Source: CAD feature listing. Evaluate the final solid. Frame: model axes, mm. Face numbers are marked on the shaded views. A direction names the side the tool comes from. Coordinates: 2 decimals unless noted, no trailing zeros. Order: outer loops, then holes, each group sorted by start corner. A loop starts at its lowest first (then second) coordinate and runs counter-clockwise, first axis right, second up. Notation, with made-up numbers: (7, -22.5) - (41, -22.5) arc R13 ccw to (41, -18.5) - close; hole circle Ø5 at (81, -24.75). An arc over 180 degrees is marked (long way). One line per question, with ' | ' between items.
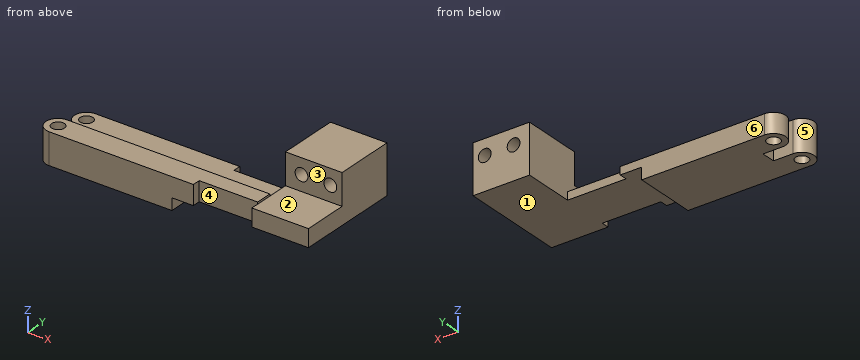
Autodesk Inventor part; units mm, degrees
ref_plane "作業平面1" through (0, 0, 5) normal (0, 0, -1) x (-1, 0, 0)
ref_plane "YZ Plane" through (0, 0, 0) normal (1, 0, 0) x (0, 1, 0)
ref_plane "XZ Plane" through (0, 0, 0) normal (0, 1, 0) x (-1, 0, 0)
sketch "スケッチ1" plane through (0, 0, 0) normal (0, 0, 1) x (1, 0, 0)
  line L0 (-3, 8) -> (3, 8)
  line L1 (3, 8) -> (3, -8)
  line L2 (3, -8) -> (-3, -8)
  line L3 (-3, -8) -> (-3, 8)
  line L4 (-3, 8) -> (3, -8) construction
  line L5 (3, 8) -> (-3, -8) construction
  line L6 (0, 8) -> (0, -8) construction
  circle A0 centre (0, 4.9) radius 1.635
  circle A1 centre (0, -4.9) radius 1.635
  line L7 (0, 4.9) -> (0, -4.9)
  line L8 (-3, 0) -> (3, 0)
  circle A2 centre (0, 4.9) radius 3.1
  circle A3 centre (0, -4.9) radius 3.1
  line L9 (3, 8) -> (52, 8)
  line L10 (52, 8) -> (52, -8)
  line L11 (52, -8) -> (3, -8)
  line L12 (0, 1.8) -> (52, 1.8)
  line L13 (0, -1.8) -> (52, -1.8)
  line L14 (5, 8) -> (5, -8)
  point P0 (0, 0)
  point P1 (0, 0)
  point P2 (3, 1.8)
  point P3 (3, -1.8)
  dimension "d0" = 3.27
  dimension "d1" = 16
  dimension "d2" = 9.8
  dimension "d3" = 6
  dimension "d11" = 2
  dimension "d12" = 47
extrude "押し出し1" add sketch "スケッチ1" along normal blind 8 contours A3 L1 L3 | L3 A3 | A3 L1
ref_plane "作業平面1" through (0, 0, 5) normal (0, 0, -1) x (-1, 0, 0)
extrude "押し出し2" add sketch "スケッチ1" against normal blind 5 from surface at 5 contours A2 L1 L3 | L3 A2 | A2 L1
extrude "押し出し3" add sketch "スケッチ1" along normal up to surface (5 mm away) contours L9 L10 L12 L14 | L12 L10 L13 L14 | L13 L10 L11 L14
extrude "押し出し4" add sketch "スケッチ1" against normal up to surface (5 mm away) from surface at 5 contours L0 L1 A2 | L9 L14 L12 L1 A2 | L9 L10 L12 L14 | L1 L12 A2
extrude "押し出し5" add sketch "スケッチ1" along normal up to surface (8 mm away) contours L14 L11 L1 A3 L13 | L13 L10 L11 L14 | L13 L1 A3 | A3 L1 L2
sketch "スケッチ2" plane through (0, 0, 0) normal (0, 1, 0) x (-1, 0, 0)
  line L0 (-52, 0) -> (-52, 5) construction
  line L1 (-52, 23) -> (-66.5, 23)
  line L2 (-66.5, 23) -> (-66.5, 0)
  line L3 (-66.5, 0) -> (-52, 0)
  line L4 (-52, 0) -> (-52, 23)
  line L5 (-66.5, 11.5) -> (-52, 11.5) construction
  line L6 (-52, 17) -> (-66.5, 17)
  line L7 (-66.5, 17) -> (-66.5, 6)
  line L8 (-66.5, 6) -> (-52, 6)
  line L9 (-52, 6) -> (-52, 17)
  line L10 (-52, 17) -> (-66.5, 6) construction
  line L11 (-66.5, 17) -> (-52, 6) construction
  circle A0 centre (-56.1, 11.5) radius 1.635
  circle A1 centre (-63.5, 11.5) radius 1.635
  line L12 (-52, 15) -> (-66.5, 15) construction
  line L13 (-52, 0) -> (-5, 0) construction
  line L14 (-52, 0) -> (-52, 5) construction
  line L15 (0, 8) -> (-52, 8) construction
  line L16 (-52, 7.5) -> (-66.5, 7.5)
  line L17 (-53.1, 6) -> (-53.1, 17)
  line L18 (-59.25, 0) -> (-59.25, 23) construction
  line L19 (-52, 15.5) -> (-66.5, 15.5)
  line L20 (-65.4, 6) -> (-65.4, 17)
  line L21 (-53.1, 7.5) -> (-53.1, 15.5)
  point P0 (-59.25, 11.5)
  point P1 (-66.5, 17)
  point P2 (-65.4, 15.5)
  point P3 (-65.4, 7.5)
  point P4 (-66.5, 15.5)
  point P5 (-66.5, 7.5)
  point P6 (-52, 7.5)
  point P7 (-52, 15.5)
  dimension "d24" = 11
  dimension "d25" = 3.27
  dimension "d26" = 4.1
  dimension "d27" = 11.5
  dimension "d32" = 3.5
  dimension "d33" = 14.5
  dimension "d36" = 3.5
  dimension "d37" = 3
  dimension "d38" = 4
extrude "押し出し7" add sketch "スケッチ2" along normal blind 30 from surface at -8
extrude "押し出し8" cut sketch "スケッチ2" against normal blind 12.5 from surface at 22 contours L4 L6 L2 L1 | L4 L19 L17 L6 | L6 L20 L19 L2 | L4 L16 L17 L19 | L17 L19 L20 L6 | L19 L20 L16 L2 | L4 L8 L17 L16 | L17 L16 L20 L19 | L16 L20 L8 L2 | L4 L3 L2 L8 | L17 L8 L20 L16 | A0 | A1
extrude "押し出し10" cut sketch "スケッチ2" along normal blind 11.6 from surface at -8 contours L4 L6 L2 L1 | L4 L19 L17 L6 | L6 L20 L19 L2 | L4 L16 L17 L19 | L17 L19 L20 L6 | L19 L20 L16 L2 | L17 L16 L20 L19
sketch "スケッチ4" plane through (0, 0, 0) normal (0, 0, -1) x (-1, 0, 0)
  circle A0 centre (0, 4.9) radius 1.635
  circle A1 centre (0, -4.9) radius 1.635
  line L0 (-52, 8) -> (-52, 9.5)
  line L1 (-52, 9.5) -> (-66.5, 9.5)
  line L2 (-66.5, -8) -> (-66.5, 9.5)
  line L3 (0, -8) -> (-66.5, -8)
  arc A2 (0, -8) -> (0, -1.8) centre (0, -4.9) ccw
  line L4 (-5, -1.8) -> (0, -1.8)
  line L5 (-5, 1.8) -> (-5, -1.8)
  line L6 (0, 1.8) -> (-5, 1.8)
  arc A3 (0, 1.8) -> (0, 8) centre (0, 4.9) ccw
  line L7 (-52, 8) -> (0, 8)
  line L8 (-52, 8) -> (-66.5, 8)
  line L9 (0, 0) -> (-66.5, 0) construction
  line L10 (-66.5, 8) -> (-31.5, 8)
  line L11 (-31.5, 8) -> (-31.5, -15)
  line L12 (-31.5, -15) -> (-66.5, -15)
  line L13 (-66.5, -15) -> (-66.5, 8)
  line L14 (-52, 8) -> (-37, 8)
  line L15 (-37, 8) -> (-37, 6)
  line L16 (-37, 6) -> (-52, 6)
  line L17 (-52, 6) -> (-52, 8)
  line L18 (-37, -8) -> (-37, -6)
  line L19 (-37, -6) -> (-52, -6)
  line L20 (-52, -6) -> (-52, -8)
  point P0 (-31.5, 8)
  point P1 (-37, 8)
  point P2 (-52, -8)
  point P3 (-37, -8)
  dimension "d41" = 35
  dimension "d42" = 23
  dimension "d43" = 15
  dimension "d44" = 2
extrude "押し出し11" cut sketch "スケッチ4" against normal blind 3 contours L8 L2 L1 L0 | L17 L16 L15 L7 L11 L3 L18 L19 L20 L2 L8 | L7 L15 L16 L17 | L3 L11 L12 L13 | L20 L19 L18 L3
extrude "押し出し12" cut sketch "スケッチ4" against normal up to surface (8 mm away) contours L7 L15 L16 L17 | L20 L19 L18 L3
sketch "スケッチ5" plane through (52, 9.5, 23) normal (0, 1, 0) x (1, 0, 0)
  circle A0 centre (11.5, 11.5) radius 1.635
  circle A1 centre (4.1, 11.5) radius 1.635
  line L0 (14.5, 20) -> (0, 20)
  line L1 (0, 0) -> (0, 20)
  line L2 (14.5, 0) -> (0, 0)
  line L3 (14.5, 20) -> (14.5, 0)
  point P0 (-52, 23)
extrude "押し出し13" add sketch "スケッチ5" along normal blind 9.6
extrude "押し出し14" cut sketch "スケッチ2" along normal through all contours L4 L6 L2 L1 | L4 L19 L17 L6 | L6 L20 L19 L2 | L17 L19 L20 L6
properties part number "link_arm_5"
(1) Material intervals for L1, parallel to Y at x = 0, z = 4.5 (3 decimals); L2, parallel to X at y = 4.9, z = 1.2 (3 decimals); L3, parallel to X at y = -4.9, z = 3.5 (3 decimals), sorted ascending. Write a range as from..to.
Taken from the geometry:
L1: y = -8..-6.535, -3.265..-1.8, 1.8..3.265, 6.535..8 | L2: x = -3.1..-1.635, 1.635..31.5 | L3: x = -3.1..-1.635, 1.635..66.5
(2) Cut plane A-A (y = 4.9). Return the cut outline in (x, z) (3 decimals).
Taken from the geometry:
outline: (-3.1, 0) - (-1.635, 0) - (-1.635, 5) - (-3.1, 5) - close; (1.635, 0) - (31.5, 0) - (31.5, 3) - (66.5, 3) - (66.5, 15.5) - (52, 15.5) - (52, 5) - (1.635, 5) - close; hole circle Ø3.27 at (56.1, 11.5); hole circle Ø3.27 at (63.5, 11.5)
(3) Pull-direction query (Y, two-part tool) for the marked faces 4, 5 and 6; classes: pulls with the +Y half, pulls with the -Y half, needs draft (parallel to the pull), parting line crosses it, or undercut.
Taken from the geometry:
face 4: pulls with the -Y half | face 5: undercut | face 6: pulls with the +Y half
(4) Cut plane C-C (x = 4). Return the cut outline in (y, z), and give its area (3 significant figures).
Taken from the geometry:
outline: (-8, 0) - (-1.8, 0) - (-1.8, 8) - (-8, 8) - close; (1.8, 0) - (8, 0) - (8, 5) - (1.8, 5) - close | area: 80.6 mm²
(5) Pin query (flat end, axial travel): P1, Ø3, axis at y = -1.5, z = 8, coming from the -X side; P2, Ø4, axis at x = 15.5, z = 3, coming from the +Y side; P3, Ø2, axis at x = 0, y = -4.9, coming from the +Z side; P4, Ø4, axis at y = 0.5, z = 3.5, coming from the -X side. Return the tip coordinate at first contact, or that it passes through.
Taken from the geometry:
P1: stops at x = -2.45 | P2: stops at y = 8 | P3: passes through | P4: stops at x = -1.96
(6) Set-up query: the marked faces 1, 2 and 3. Return all of +Z, -Z, +X, -X, +Y, -Y with unobstructed straight access to the full face (end or side cutting, diameter ignored); none if empty.
Taken from the geometry:
face 1: -Z, +X, +Y, -Y | face 2: +Z, +X, -Y | face 3: +Z, +X, -X, -Y
(7) Cut plane D-D (y = -4.9). Return the cut outline in (x, z) (3 decimals).
Taken from the geometry:
outline: (-3.1, 0) - (-1.635, 0) - (-1.635, 8) - (-3.1, 8) - close; (1.635, 0) - (31.5, 0) - (31.5, 3) - (66.5, 3) - (66.5, 7.5) - (52, 7.5) - (52, 8) - (1.635, 8) - close
(8) Cut plane B-B (z = 4.25). Return the cut outline in (x, y) (3 decimals), and give its area (3 significant figures).
Taken from the geometry:
outline: (0, -8) - (37, -8) - (37, -6) - (52, -6) - (52, -8) - (66.5, -8) - (66.5, 19.1) - (52, 19.1) - (52, 6) - (37, 6) - (37, 8) - (0, 8) arc R3.1 ccw to (0, 1.8) - (5, 1.8) - (5, -1.8) - (0, -1.8) arc R3.1 ccw to start; hole circle Ø3.27 at (0, -4.9); hole circle Ø3.27 at (0, 4.9) | area: 1,160 mm²
